```python
from build123d import *

# Parameters (mm, degrees)
F0_W     = 7
F0_H     = 7
F1_DEPTH = 0.5
F2_R     = 3.5
F2_R_2   = 1.5
F3_DEPTH = 6
F4_SIZE2 = 1
F4_SIZE  = 0.15


with BuildPart() as f1:
    # F0 (on Top) → F1 (new body)
    with BuildSketch(Plane.XY):
        with Locations((3.5, 3.5)):
            Rectangle(F0_W, F0_H)
    extrude(amount=F1_DEPTH)

    # F2 (on face) → F3 (join)
    with BuildSketch(Plane.XY.offset(0.5)):
        with Locations((3.5, 3.5)):
            Circle(F2_R)
        with Locations((3.5, 3.5)):
            Circle(F2_R_2, mode=Mode.SUBTRACT)
    extrude(amount=F3_DEPTH)

    # F4
    f4_edges = [f1.edges().sort_by_distance(p)[0] for p in [
        (2, 3.5, 6.5),
    ]]
    chamfer(f4_edges, length=F4_SIZE, length2=F4_SIZE2)


solid = f1.part
```
The listing builds one solid part. Answer for the finished solid, in the listing's coordinates (mm). A direction names the side the tool comes from. Coordinates: 2 decimals unless noted, no trailing zeros. Loops run counter-clockwise (first coordinate to the right, second up) from the corner with the lowest first, then second, coordinate; pieces in that order, holes last. Notation, with made-up numbers: M 65.25,45 L 90.25,45 A18 cw 90.25,60 Z; hole C 66.25,17 d9. An arc over 180 degrees is marked long. Answer as a JSON object with one key per item and string values. Group by question number.
Item 1: This flat-tipped pin is pushed along its axis until it touches: P1, Ø1, axis at x = 4, y = 4, coming from the +Z side. Where does it stop, or does it pass through?
Item 2: Section B-B (y = 1.5) is taken. Write down the section's boundary in (x, z).
Item 3: Consider L1, parallel to Y at x = 3.5, z = 2.15; L2, parallel to Z at x = 0.5, y = 1; L3, parallel to Y at x = 4.5, z = 2.5. Determine where each line is inside the solid, lowest interval first.
Item 4: Section A-A (x = 0.75) is taken. Write down the section's boundary in (y, z), and give its area (3 significant figures).
Item 5: Section C-C (z = 4) is taken. Write down the section's boundary in (x, y).
Item 6: Determine the mould class of faces 4 (the face through (0.7, 6.2, 0.5)), 5 (the face through (3, 4, 0.5)), 6 (the face through (5.115, 0.395, 3.458)), 7 (the face through (4.886, 2.925, 2.965)) for opening direction Y: +Y half, -Y half, draft (parallel to the pull), parting line (faces both ways), or undercut.
Item 7: Which of the six approach directions +Z, -Z, +X, -X, +Y, -Y give full straight-line access (tool end or side, diameter ignored) to faces 1 (the face through (6.1, 6.3, 0.5)), 2 (the face through (6.3, 0.7, 0.5)), 3 (the face through (0.7, 0.9, 0.5))?
Solved:
{
 "1": {"P1": "stops at z = 0.5"},
 "2": {"outline": "M 0,0 L 7,0 L 7,0.5 L 6.37,0.5 L 6.37,6.5 L 0.63,6.5 L 0.63,0.5 L 0,0.5 Z"},
 "3": {"L1": "y = 0 to 2, 5 to 7", "L2": "z = 0 to 0.5", "L3": "y = 0.15 to 2.38, 4.62 to 6.85"},
 "4": {"outline": "M 0,0 L 7,0 L 7,0.5 L 5.67,0.5 L 5.67,6.5 L 1.33,6.5 L 1.33,0.5 L 0,0.5 Z", "area": "29.5 mm2"},
 "5": {"outline": "C 3.5,3.5 d7; hole C 3.5,3.5 d3"},
 "6": {"face 4": "draft", "face 5": "undercut", "face 6": "parting line", "face 7": "undercut"},
 "7": {"face 1": "+Z, +X, +Y", "face 2": "+Z, +X, -Y", "face 3": "+Z, -X, -Y"}
}
